Work out the finished part from the listing and answer in its coordinate system (mm). A direction names the side the tool comes from. Coordinates: 2 decimals unless noted, no trailing zeros. Order: outer loops, then holes, each group sorted by start corner. A loop starts at its lowest first (then second) coordinate and runs counter-clockwise, first axis right, second up. Notation, with made-up numbers: M -31,-10 L 3,-10 A26 ccw 3,25 Z; hole C 45,-10.5 d8. An arc over 180 degrees is marked long. Answer in a Markdown table with one row per item. Add a question column.
Item 1: Consider line 1 (Y direction, x = 68.3, z = 0) (3 decimals); line 2 (X direction, y = 3, z = 19.05); line 3 (X direction, y = 0, z = -22). Determine where each line is inside the solid, lowest interval first. Write a range as from..to.
Item 2: The part is cut by section A-A (z = 19.05). Write down the section's boundary in (x, y) (3 decimals).
Item 3: The part is cut by section B-B (z = -19.05). Write down the section's boundary in (x, y) (3 decimals), then the cut area to 3 significant figures.
Item 4: Flat-ended cylindrical pins translate along their axes: pin 1 Ø12 at (x, y) = (21.5, 3) entering from -Z; pin 2 Ø6 at (x, y) = (12.7, 14.3) entering from -Z; pin 3 Ø2.5 at (x, z) = (-23.5, -1) entering from +Y. Find the tip coordinate at first contact, or state that the pin passes through.
Item 5: The part is cut by section C-C (x = -13). Write down the section's boundary in (y, z), then the cut area to 3 significant figures.
Item 6: The mould has two halves that part along Y. Classify faces 5 (the face through (34, -22.225, 0)), 6 (the face through (48.874, -0.219, -16.628)), 7 (the face through (-24, 8.585, 0)): released by +Y, released by -Y, zero draft, split by the parting line, or undercut.
Item 7: The part is cut by section D-D (x = 34). Write down the section's boundary in (y, z) (3 decimals), then the cut area to 3 significant figures.
Item 8: Which of the six approach directions +Z, -Z, +X, -X, +Y, -Y give full straight-line access (tool end or side, diameter ignored) to faces 1 (the face through (69.723, 10, 0)), 2 (the face through (54, 0, -11.176)), 3 (the face through (61.12, 3.02, -26.4)), 4 (the face through (-12.77, 10.23, -1.34))?
from build123d import *

# Parameters (mm, degrees)
SKETCH1_W          = 50.8
SKETCH1_H          = 44.45
EXTRUDE1_DEPTH     = 69.723
SKETCH5_R          = 17.4625
EXTRUDE2_DEPTH     = 5.969
SKETCH6_W          = 10.31875
SKETCH6_H          = 20.828
CUT_EXTRUDE4_DEPTH = 30.48
SKETCH13_R         = 7.874
EXTRUDE3_DEPTH     = 2.54
HOLE1_D            = 7.1374
HOLE1_DEPTH        = 69.723
HOLE2_D            = 8.7376
HOLE2_DEPTH        = 44.45
SKETCH18_R         = 7.874
EXTRUDE4_DEPTH     = 2.54


with BuildPart() as part:
    # Sketch1 → Extrude1 (new body)
    with BuildSketch(Plane(origin=(0, 0, 0), x_dir=(0, 0, -1), z_dir=(1, 0, 0))):
        Rectangle(SKETCH1_W, SKETCH1_H)
    extrude(amount=EXTRUDE1_DEPTH)

    # S2D0002 → Cut-Revolve1 (revolve, cut)
    with BuildSketch(Plane(origin=(0, 14.3002, 0), x_dir=(-1, 0, 0), z_dir=(0, 1, 0)), mode=Mode.PRIVATE) as cut_revolve1_sk:
        Polygon((-18.8849, -25.146), (-22.225, -25.146), (-22.225, -25.4), (-12.7, -25.4), (-12.7, -11.176), (-17.6784, -11.176), (-17.6784, -21.929393135), (-18.342306865, -22.5933), align=None)
    revolve(cut_revolve1_sk.sketch.rotate(Axis((12.7, 14.3002, -19.13842003), (0, 0, 1)), 180), axis=Axis((12.7, 14.3002, -19.13842003), (0, 0, 1)), mode=Mode.SUBTRACT)  # turned: the seam where the file's is

    # Sketch3 → Cut-Revolve2 (revolve, cut)
    with BuildSketch(Plane(origin=(41.148, 0, -25.146), x_dir=(1, 0, 0), z_dir=(0, 1, 0))):
        Polygon((18.8849, 0), (22.225, 0), (22.225, 0.254), (12.7, 0.254), (12.7, -13.97), (17.6784, -13.97), (17.6784, -3.216606865), (18.342306865, -2.5527), align=None)
    revolve(axis=Axis((53.848, 0, -3.189624441), (0, 0, -1)), mode=Mode.SUBTRACT)

    # Sketch4 → Cut-Revolve3 (revolve, cut)
    with BuildSketch(Plane(origin=(53.975, 0, 0), x_dir=(0, -1, 0), z_dir=(0, 0, 1)), mode=Mode.PRIVATE) as cut_revolve3_sk:
        Polygon((6.1849, 12.7), (9.525, 12.7), (9.525, 15.748), (0, 15.748), (0, 1.3462), (4.9784, 1.3462), (4.9784, 9.483393135), (5.642306865, 10.1473), align=None)
    revolve(cut_revolve3_sk.sketch.rotate(Axis((38.879609832, 0, 0), (1, 0, 0)), 270), axis=Axis((38.879609832, 0, 0), (1, 0, 0)), mode=Mode.SUBTRACT)  # turned: the seam where the file's is

    # Sketch5 → Extrude2 (add)
    with BuildSketch(Plane.ZY):
        Circle(SKETCH5_R)
    extrude(amount=EXTRUDE2_DEPTH)

    # Sketch6 → Revolve1 (revolve)
    with BuildSketch(Plane(origin=(0, 0, 0), x_dir=(0, 0, 1), z_dir=(0, -1, 0)), mode=Mode.PRIVATE) as revolve1_sk:
        with Locations((-5.159375, 16.383)):
            Rectangle(SKETCH6_W, SKETCH6_H)
    revolve(revolve1_sk.sketch.rotate(Axis((5.754582971, 0, 0), (-1, 0, 0)), 180), axis=Axis((5.754582971, 0, 0), (-1, 0, 0)))  # turned: the seam where the file's is

    # S2D0001 → Cut-Revolve4 (revolve, cut)
    with BuildSketch(Plane(origin=(-18.511260017, 3.2639, 0), x_dir=(0, 1, 0), z_dir=(0, 0, 1)), mode=Mode.PRIVATE) as cut_revolve4_sk:
        Polygon((0, 6.35), (0, -6.522460017), (-3.2639, -6.522460017), (-3.2639, 8.285739983), (1.1176, 8.285739983), align=None)
    revolve(cut_revolve4_sk.sketch.rotate(Axis((0, 0, 0), (-1, 0, 0)), 270), axis=Axis((0, 0, 0), (-1, 0, 0)), mode=Mode.SUBTRACT)  # turned: the seam where the file's is

    # Sketch8 → Cut-Revolve5 (revolve, cut)
    with BuildSketch(Plane(origin=(0, 0, 0), x_dir=(0, 0, -1), z_dir=(0, 1, 0)), mode=Mode.PRIVATE) as cut_revolve5_sk:
        with BuildLine():
            Line((-10.31875, 19.3802), (-10.033, 20.1422))
            Line((-10.033, 20.1422), (-10.033, 25.781))
            ThreePointArc((-10.033, 25.781), (-9.932678675, 26.324796865), (-9.644922533, 26.797))
            Line((-9.644922533, 26.797), (-10.31875, 26.797))
            Line((-10.31875, 26.797), (-10.31875, 19.3802))
        make_face()
    revolve(cut_revolve5_sk.sketch.rotate(Axis((-12.65936, 0, 0), (-1, 0, 0)), 180), axis=Axis((-12.65936, 0, 0), (-1, 0, 0)), mode=Mode.SUBTRACT)  # turned: the seam where the file's is

    # Sketch12 → Cut-Extrude4 (cut, symmetric)
    with BuildSketch(Plane(origin=(0, 0, 0), x_dir=(0, -1, 0), z_dir=(0, 0, -1))):
        Polygon((8.5852, 26.797), (8.5852, 21.844), (10.033, 20.3962), (10.033, 26.797), align=None)
        Polygon((-8.5852, 26.797), (-8.5852, 21.844), (-10.033, 20.3962), (-10.033, 26.797), align=None)
    extrude(amount=CUT_EXTRUDE4_DEPTH, both=True, mode=Mode.SUBTRACT)

    # Sketch13 → Extrude3 (add)
    with BuildSketch(Plane(origin=(0, 0, -25.146), x_dir=(-1, 0, 0), z_dir=(0, 0, -1))):
        with Locations(Location((-53.848, 0, 0), (0, 0, 180))):  # turned: the seam where the file's is
            Circle(SKETCH13_R)
    extrude(amount=EXTRUDE3_DEPTH)

    # Hole1
    with Locations(Plane.ZY):
        with Locations((-19.05, -15.875), (19.05, 15.875)):
            Hole(HOLE1_D / 2, depth=HOLE1_DEPTH)

    # Hole2
    with Locations(Plane(origin=(0, 22.225, 0), x_dir=(-1, 0, 0), z_dir=(0, 1, 0))):
        with Locations((-26.797, -19.05), (-26.797, 19.05)):
            Hole(HOLE2_D / 2, depth=HOLE2_DEPTH)

    # Sketch18 → Extrude4 (add)
    with BuildSketch(Plane(origin=(66.675, 0, 0), x_dir=(0, 0, -1), z_dir=(1, 0, 0))):
        with Locations(Location((0, 0, 0), (0, 0, 180))):  # turned: the seam where the file's is
            Circle(SKETCH18_R)
    extrude(amount=EXTRUDE4_DEPTH)


solid = part.part
Reply:
| question | item | result |
|---|---|---|
| 1 | line 1 | y = -22.225..-9.525, -7.874..7.874, 9.525..22.225 |
| 1 | line 2 | x = 0..22.43, 31.17..69.72 |
| 1 | line 3 | x = 0..23.57, 30.02..48.8, 58.9..69.72 |
| 2 | outline | M 0,-22.225 L 22.428,-22.225 L 22.428,12.306 L 0,12.306 Z; M 0,19.444 L 22.428,19.444 L 22.428,22.225 L 0,22.225 Z; M 31.166,-22.225 L 69.723,-22.225 L 69.723,12.306 L 31.166,12.306 Z; M 31.166,19.444 L 69.723,19.444 L 69.723,22.225 L 31.166,22.225 Z |
| 3 | outline | M 0,-22.225 L 22.428,-22.225 L 22.428,-19.444 L 0,-19.444 Z; M 0,-12.306 L 22.428,-12.306 L 22.428,22.225 L 0,22.225 Z; M 31.166,-22.225 L 69.723,-22.225 L 69.723,-19.444 L 31.166,-19.444 Z; M 31.166,-12.306 L 69.723,-12.306 L 69.723,22.225 L 31.166,22.225 Z; hole C 12.7,14.3 d9.957; hole C 53.848,0 d9.957 |
| 3 | area | 2,120 mm2 |
| 4 | pin 1 | stops at z = -25.4 |
| 4 | pin 2 | stops at z = -11.18 |
| 4 | pin 3 | stops at y = 8.59 |
| 5 | outline | C 0,0 d20.64; hole C 0,0 d6.53 |
| 5 | area | 301 mm2 |
| 6 | face 5 | released by -Y |
| 6 | face 6 | undercut |
| 6 | face 7 | released by +Y |
| 7 | outline | M -22.225,-25.4 L 22.225,-25.4 L 22.225,25.4 L -22.225,25.4 Z; hole C -15.875,-19.05 d7.137; hole C 15.875,19.05 d7.137 |
| 7 | area | 2,180 mm2 |
| 8 | face 1 | +Z, -Z, +X, +Y, -Y |
| 8 | face 2 | none |
| 8 | face 3 | -Z |
| 8 | face 4 | -X |
